Verification items for the finished model (mm, model axes). Round coordinates to 2 decimals unless told otherwise and drop trailing zeros. Loops run counter-clockwise (first coordinate to the right, second up) from the corner with the lowest first, then second, coordinate; pieces in that order, holes last. Notation, with made-up numbers: (54, 57.5) - (90, 57.5) arc R33 ccw to (90, 92.5) - close; hole circle Ø8 at (9.5, 47). An arc over 180 degrees is marked (long way). Use CSV: the item, a comma, the result in double quotes.
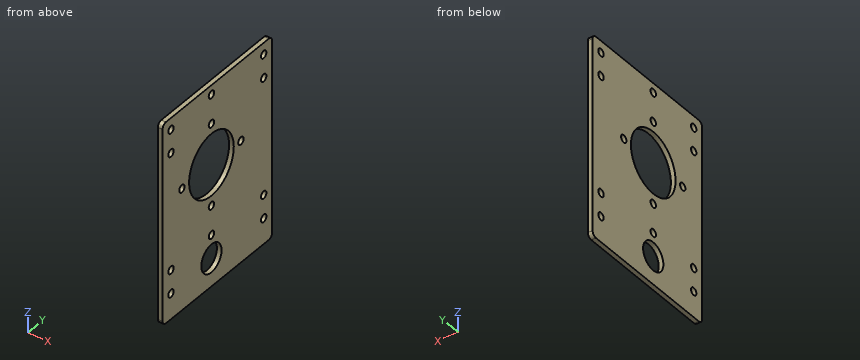
Autodesk Inventor part; units mm, degrees
ref_plane "YZ Plane" through (0, 0, 0) normal (1, 0, 0) x (0, 1, 0)
ref_plane "XZ Plane" through (0, 0, 0) normal (0, 1, 0) x (-1, 0, 0)
ref_plane "XY Plane" through (0, 0, 0) normal (0, 0, 1) x (1, 0, 0)
sketch "Sketch1" plane through (0, 0, 0) normal (1, 0, 0) x (0, 1, 0)
  circle A0 centre (0, 0) radius 13.25
  line L0 (36, -46) -> (36, 34)
  line L1 (36, 34) -> (-29, 34)
  line L2 (-29, 34) -> (-29, -46)
  line L3 (-29, -46) -> (36, -46)
  point P0 (0, -17.5)
  point P1 (17.5, 0)
  point P2 (0, 17.5)
  point P3 (-17.5, 0)
  point P4 (0, -30)
  point P5 (0, 30)
  point P6 (31, -41)
  point P7 (31, 29)
  point P8 (-24, 29)
  point P9 (-24, -41)
  dimension "d0" = 26.5
  dimension "d1" = 17.5
  dimension "d4" = 360
  dimension "d6" = 30
  dimension "d9" = 360
  dimension "d15" = 5
  dimension "d16" = 5
  dimension "d17" = 80
  dimension "d18" = 65
  dimension "d28" = 5
  dimension "d29" = 55
  dimension "d30" = 55
extrude "Extrusion1" add sketch "Sketch1" along normal blind 2
hole "Hole1" at (0, 0, -17.5) at (0, 17.5, 0) at (0, 0, 17.5) at (0, -17.5, 0) at (0, 0, -30) at (0, 0, 30) at (0, 31, -41) at (0, 31, 29) at (0, -24, 29) at (0, -24, -41) direction (1, 0, 0) diameter 3.2 depth 43.75 tip angle 118
sketch "Sketch2" plane through (0, 0, 0) normal (-1, 0, 0) x (0, 0, 1)
  circle A0 centre (-40, 0) radius 6
  line L0 (-46, 36) -> (34, 36)
  line L1 (-46, 36) -> (-52, 36)
  line L2 (-52, 36) -> (-52, -29)
  line L3 (-52, -29) -> (-46, -29)
  line L4 (-46, -29) -> (-46, 36)
  point P0 (0, 0)
  point P1 (0, 25.1294)
  point P2 (0, -32.6005)
  dimension "d31" = 40
  dimension "d32" = 12
  dimension "d33" = 6
extrude "Extrusion2" add sketch "Sketch2" against normal blind 2 contours L4 L3 L2 L1
extrude "Extrusion3" cut sketch "Sketch2" against normal blind 2 contours A0
sketch "Sketch3" plane through (2, 0, 0) normal (1, 0, 0) x (0, 0, -1)
  circle A0 centre (41, 31) radius 1.6
  circle A1 centre (-29, 31) radius 1.6
  circle A2 centre (-29, -24) radius 1.6
  circle A3 centre (41, -24) radius 1.6
  point P0 (0, 0)
  point P1 (-19, 31)
  point P2 (31, 31)
  point P3 (-19, -24)
  point P4 (31, -24)
  dimension "d38" = 10
  dimension "d39" = 10
  dimension "d40" = 10
  dimension "d41" = 10
hole "Hole2" at (2, 31, 19) at (2, 31, -31) at (2, -24, 19) at (2, -24, -31) direction (-1, 0, 0) diameter 3.2 depth 43.75 tip angle 118
fillet "Fillet1" radius 2 4 edges at (1, 36, 34) (1, 36, -52) (1, -29, -52) (1, -29, 34)
properties part number "motor" material "アルミニウム 6061"
1) Cross-section at B-B, the plane y = -24. Record the cut outline in (x, z).
Returned:
outline,"(0, -52) - (2, -52) - (2, -42.6) - (0, -42.6) - close; (0, -39.4) - (2, -39.4) - (2, -32.6) - (0, -32.6) - close; (0, -29.4) - (2, -29.4) - (2, 17.4) - (0, 17.4) - close; (0, 20.6) - (2, 20.6) - (2, 27.4) - (0, 27.4) - close; (0, 30.6) - (2, 30.6) - (2, 34) - (0, 34) - close"
2) Cross-section at D-D, the plane y = 0. Record the cut outline in (x, z), then the cut area to 3 significant figures.
Returned:
outline,"(0, -52) - (2, -52) - (2, -46) - (0, -46) - close; (0, -34) - (2, -34) - (2, -31.6) - (0, -31.6) - close; (0, -28.4) - (2, -28.4) - (2, -19.1) - (0, -19.1) - close; (0, -15.9) - (2, -15.9) - (2, -13.25) - (0, -13.25) - close; (0, 13.25) - (2, 13.25) - (2, 15.9) - (0, 15.9) - close; (0, 19.1) - (2, 19.1) - (2, 28.4) - (0, 28.4) - close; (0, 31.6) - (2, 31.6) - (2, 34) - (0, 34) - close"
area,"69.4 mm²"
3) Thickness scan on probe 1 along Z at (x, y) = (0.5, -24); probe 2 along Y at (x, z) = (0.5, -42); probe 3 along Z at (x, y) = (0.1, 5.5). Record the ranges inside material, lowest first. Write a range as [from, to].
Returned:
probe 1,"z = [-52, -42.6], [-39.4, -32.6], [-29.4, 17.4], [20.6, 27.4], [30.6, 34]"
probe 2,"y = [-29, -25.25], [-22.75, -5.66], [5.66, 29.75], [32.25, 36]"
probe 3,"z = [-52, -42.4], [-37.6, -12.05], [12.05, 34]"
4) Gauge pin test, flat end, axial feed: pin 1 Ø2.5 at (y, z) = (-24, -31) entering from +X. Record the tip position at first contact, or that the pin passes through.
Returned:
pin 1,"passes through"
5) Cross-section at C-C, the plane x = 0.8. Count the separate pieces of the cut face and the enclosed holes in it, then the cut area to 3 significant figures.
Returned:
separate pieces,"1"
enclosed holes,"16"
area,"4,810 mm²"
6) Cross-section at A-A, the plane z = 0. Record the cut outline in (x, y).
Returned:
outline,"(0, -29) - (2, -29) - (2, -19.1) - (0, -19.1) - close; (0, -15.9) - (2, -15.9) - (2, -13.25) - (0, -13.25) - close; (0, 13.25) - (2, 13.25) - (2, 15.9) - (0, 15.9) - close; (0, 19.1) - (2, 19.1) - (2, 36) - (0, 36) - close"
